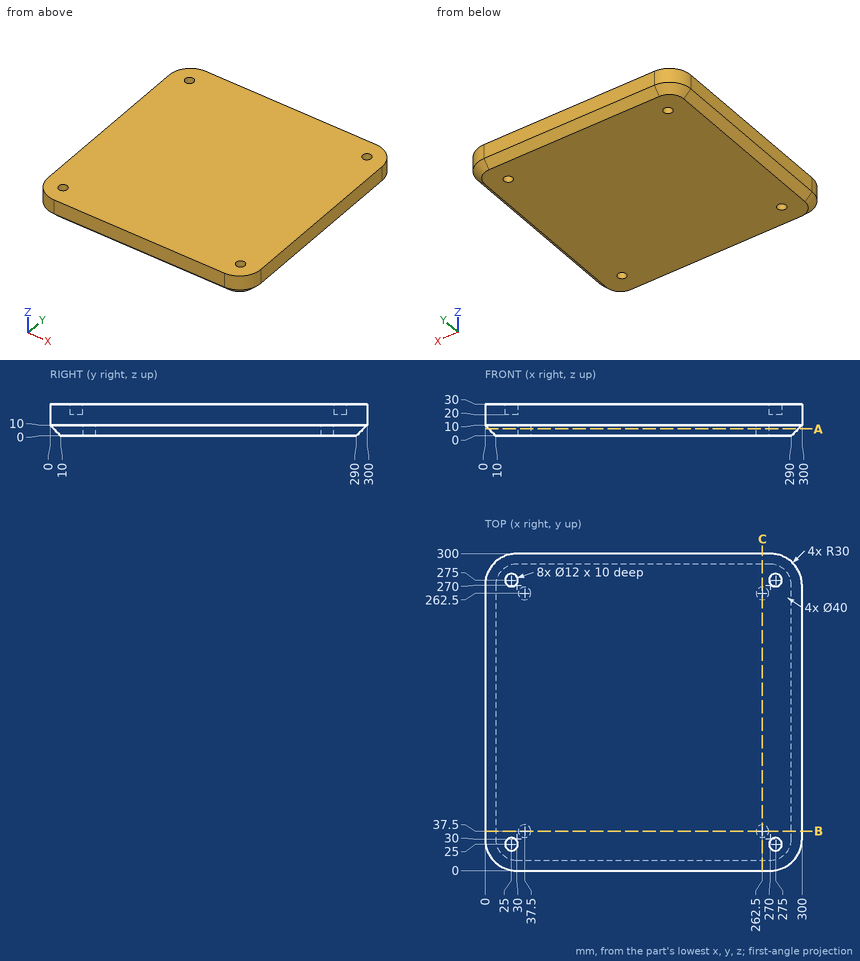
Answer from the drawing. Dimensions are ordinates in mm from the lowest x, y and z of the part. Coordinates: 2 decimals unless noted, no trailing zeros. Write each loop counter-clockwise with the first axis right and the second up, starting at its lowest first coordinate (ties: lowest second). Pieces come first, ordered by that corner, then holes. Notation, with made-up numbers: (-15.75, -34) - (16.25, -34) arc R31 cw to (16.25, -9) - close; hole circle Ø8 at (22.5, 10). An arc over 180 degrees is marked (long way). Return JSON: item names as keys, results as strings.
1. Each of these flat-tipped pins is pushed along its axis until it touches: pin 1 Ø6 at (x, y) = (275.5, 277.5) entering from +Z; pin 2 Ø7 at (x, y) = (37.5, 262.5) entering from -Z. Where does it stop, or does it pass through?
Final values:
{"pin 1": "z = 20", "pin 2": "z = 10"}
2. Consider line 1 along X through (y, z) = (275, 25.5); line 2 along Y through (x, z) = (37.5, 2.25). Determine where each line is inside the solid, lowest interval first.
Final values:
{"line 1": "0.42 to 19, 31 to 269, 281 to 299.58", "line 2": "7.75 to 31.5, 43.5 to 256.5, 268.5 to 292.25"}
3. The part is cut by section A-A on z = 6.5. Determine the outline of the cut face in (x, y).
Final values:
{"outline": "(3.5, 30) arc R26.5 ccw to (30, 3.5) - (270, 3.5) arc R26.5 ccw to (296.5, 30) - (296.5, 270) arc R26.5 ccw to (270, 296.5) - (30, 296.5) arc R26.5 ccw to (3.5, 270) - close; hole circle Ø12 at (37.5, 37.5); hole circle Ø12 at (37.5, 262.5); hole circle Ø12 at (262.5, 37.5); hole circle Ø12 at (262.5, 262.5)"}
4. The part is cut by section B-B on y = 37.5. Determine the outline of the cut face in (x, z), then the cut area to 3 significant figures.
Final values:
{"outline": "(0, 10) - (10, 0) - (31.5, 0) - (31.5, 10) - (43.5, 10) - (43.5, 0) - (256.5, 0) - (256.5, 10) - (268.5, 10) - (268.5, 0) - (290, 0) - (300, 10) - (300, 30) - (0, 30) - close", "area": "8,660 mm^2"}
